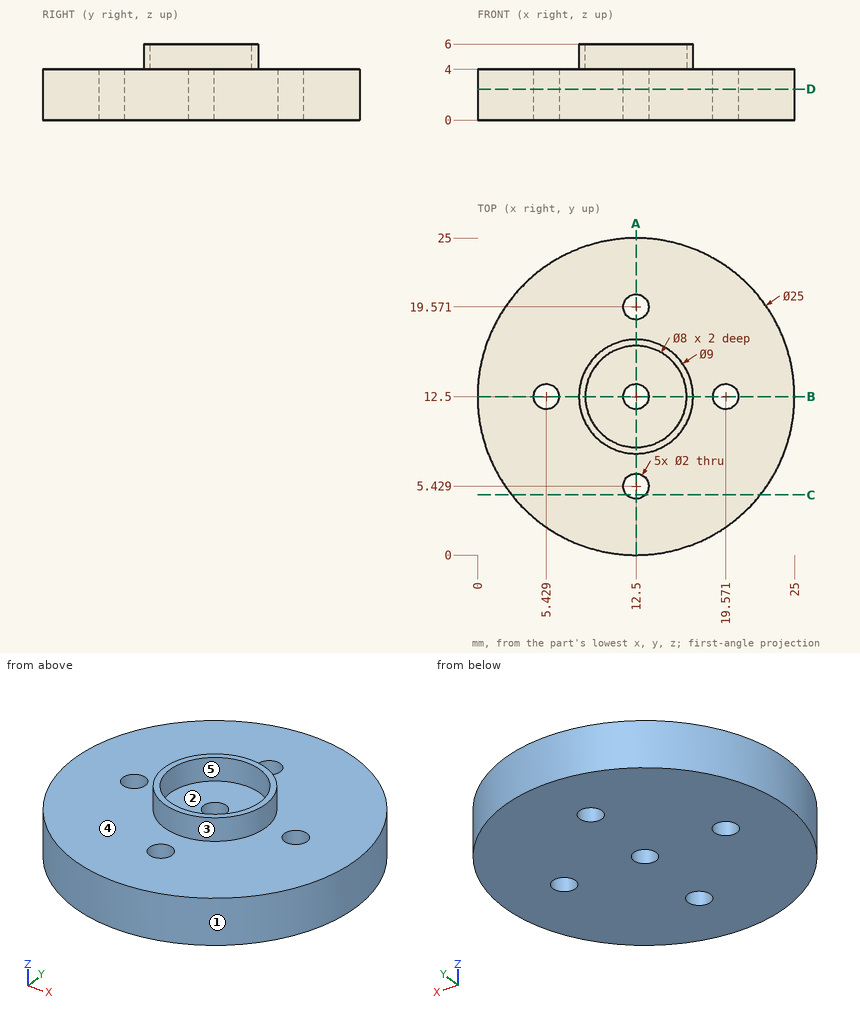
Source: three-view drawing plus pictorial views. Frame: mm from the lowest corner of the part. A direction names the side the tool comes from. Round coordinates to 2 decimals unless told otherwise and drop trailing zeros. Order: outer loops, then holes, each group sorted by start corner. A loop starts at its lowest first (then second) coordinate and runs counter-clockwise, first axis right, second up. Notation, with made-up numbers: (82, -8.75) -> (121, -8.75) arc R19 cw to (121, 28.25) -> close; hole circle Ø2 at (48.25, 65.25). An arc over 180 degrees is marked (long way). Use one line per item in the form item = value.
(1) Section D-D on z = 2.45. Return loops of the section in (x, y).
Results list:
outline = circle Ø25 at (12.5, 12.5); hole circle Ø2 at (5.43, 12.5); hole circle Ø2 at (12.5, 5.43); hole circle Ø2 at (12.5, 12.5); hole circle Ø2 at (12.5, 19.57); hole circle Ø2 at (19.57, 12.5)
(2) Access query for the marked faces 1 and 2. Directions: +Z, -Z, +X, -X, +Y, -Y. A direction counts if a zero-diameter tool reaches every point of the face in a straight line with its end or side. Return the directions, or none.
Results list:
face_1 = +Z, -Z
face_2 = +Z
(3) First-contact query: pin 1 Ø7 at (x, y) = (12.5, 12.5) entering from +Z; pin 2 Ø1.5 at (x, z) = (8, 3) entering from -Y; pin 3 Ø1.5 at (x, z) = (10, 3) entering from -Y; pin 4 Ø1.6 at (x, y) = (19.57, 12.5) entering from -Z. Flat tips, straight axial feed; report the tip coordinate or a pass-through.
Results list:
pin_1 = 4
pin_2 = 0.58
pin_3 = 0.12
pin_4 = through
(4) Section A-A on x = 12.5. Return loops of the section in (y, z).
Results list:
outline = (0, 0) -> (4.43, 0) -> (4.43, 4) -> (0, 4) -> close; (6.43, 0) -> (11.5, 0) -> (11.5, 4) -> (8.5, 4) -> (8.5, 6) -> (8, 6) -> (8, 4) -> (6.43, 4) -> close; (13.5, 0) -> (18.57, 0) -> (18.57, 4) -> (17, 4) -> (17, 6) -> (16.5, 6) -> (16.5, 4) -> (13.5, 4) -> close; (20.57, 0) -> (25, 0) -> (25, 4) -> (20.57, 4) -> close
(5) Ray query, probe 1 along Y at (x, z) = (12.5, 3); probe 2 along Y at (x, z) = (12, 1.95) (3 decimals); probe 3 along Z at (x, y) = (10.75, 17.75). Return the intervals inside material, ascending. Write a range as [from, to].
Results list:
probe_1 = [0, 4.43], [6.43, 11.5], [13.5, 18.57], [20.57, 25]
probe_2 = [0.01, 4.563], [6.295, 11.634], [13.366, 18.705], [20.437, 24.99]
probe_3 = [0, 4]
(6) Section C-C on y = 4.75. Return loops of the section in (x, z).
Results list:
outline = (2.69, 0) -> (11.77, 0) -> (11.77, 4) -> (2.69, 4) -> close; (13.23, 0) -> (22.31, 0) -> (22.31, 4) -> (13.23, 4) -> close
(7) Draft query along Y for the marked faces 3, 4 and 5. Return one class per face: pulls with the +Y half, pulls with the -Y half, needs draft (parallel to the pull), parting line crosses it, or undercut.
Results list:
face_3 = parting line crosses it
face_4 = needs draft
face_5 = undercut
